```python
from build123d import *

# Parameters (mm, degrees)
SKETCH_2_W           = 70
SKETCH_2_H           = 60
EXTRUDE_2_DEPTH      = 40
SKETCH_3_W           = 40.7
SKETCH_3_H           = 20.5
CUT_EXTRUDE_1_DEPTH  = 28
SKETCH_4_W           = 14.65
SKETCH_4_H           = 20.5
EXTRUDE_3_DEPTH      = 28
SKETCH_15_W          = 40.7
SKETCH_15_H          = 40.25
CUT_EXTRUDE_6_DEPTH  = 28
SKETCH_16_W          = 14.65
SKETCH_16_H          = 20.204149113
CUT_EXTRUDE_7_DEPTH  = 40
M3X0_5_2_D           = 2.5
CUT_EXTRUDE_8_DEPTH  = 3
CUT_EXTRUDE_9_DEPTH  = 3
CUT_EXTRUDE_10_DEPTH = 6
M3X0_5_3_D           = 2.5
M3X0_5_3_DEPTH       = 40
M3X0_5_3_TIP         = 0.751075774
CUT_EXTRUDE_12_DEPTH = 5


with BuildPart() as part:
    # ｽｹｯﾁ2 → ﾎﾞｽ - 押し出し2 (new body)
    with BuildSketch(Plane.XY):
        Rectangle(SKETCH_2_W, SKETCH_2_H)
    extrude(amount=EXTRUDE_2_DEPTH)

    # ｽｹｯﾁ3 → ｶｯﾄ - 押し出し1 (cut)
    with BuildSketch(Plane.XY):
        Rectangle(SKETCH_3_W, SKETCH_3_H)
    extrude(amount=CUT_EXTRUDE_1_DEPTH, mode=Mode.SUBTRACT)

    # ｽｹｯﾁ4 → ﾎﾞｽ - 押し出し3 (add)
    with BuildSketch(Plane.XY):
        with Locations((27.675, 0)):
            Rectangle(SKETCH_4_W, SKETCH_4_H)
    extrude(amount=EXTRUDE_3_DEPTH)

    # ｽｹｯﾁ15 → ｶｯﾄ - 押し出し6 (cut)
    with BuildSketch(Plane.XY):
        with Locations((0, -9.875)):
            Rectangle(SKETCH_15_W, SKETCH_15_H)
    extrude(amount=CUT_EXTRUDE_6_DEPTH, mode=Mode.SUBTRACT)

    # ｽｹｯﾁ16 → ｶｯﾄ - 押し出し7 (cut)
    with BuildSketch(Plane(origin=(0, -30, 0), x_dir=(-1, 0, 0), z_dir=(0, -1, 0))):
        with Locations((-27.675, -17.897925444)):
            Rectangle(SKETCH_16_W, SKETCH_16_H)
    extrude(amount=-CUT_EXTRUDE_7_DEPTH, mode=Mode.SUBTRACT)

    # M3x0.5 ねじ穴2 (through all)
    with Locations(Plane(origin=(0, 0, 0), x_dir=(-1, 0, 0), z_dir=(0, 0, -1))):
        with Locations((24.85, 5), (24.85, -5)):
            m3x0_5_2 = Hole(M3X0_5_2_D / 2)

    # ﾐﾗｰ1: M3x0.5 ねじ穴2 across plane
    add(m3x0_5_2.mirror(Plane(origin=(0, 0, 0), x_dir=(0, 0, 1), z_dir=(1, 0, 0))), mode=Mode.SUBTRACT)

    # ｽｹｯﾁ17 → ｶｯﾄ - 押し出し8 (cut)
    with BuildSketch(Plane.XY.offset(40)):
        Polygon((-24.85, 8.290896534), (-27.7, 6.645448267), (-27.7, 3.354551733), (-24.85, 1.709103466), (-22, 3.354551733), (-22, 6.645448267), align=None)
        Polygon((-22, -6.645448267), (-22, -3.354551733), (-24.85, -1.709103466), (-27.7, -3.354551733), (-27.7, -6.645448267), (-24.85, -8.290896534), align=None)
    extrude(amount=-CUT_EXTRUDE_8_DEPTH, mode=Mode.SUBTRACT)

    # ｽｹｯﾁ18 → ｶｯﾄ - 押し出し9 (cut)
    with BuildSketch(Plane.XY.offset(7.795850887)):
        Polygon((27.7, 3.354551733), (27.7, 6.645448267), (24.85, 8.290896534), (22, 6.645448267), (22, 3.354551733), (24.85, 1.709103466), align=None)
        Polygon((27.7, -6.645448267), (27.7, -3.354551733), (24.85, -1.709103466), (22, -3.354551733), (22, -6.645448267), (24.85, -8.290896534), align=None)
    extrude(amount=-CUT_EXTRUDE_9_DEPTH, mode=Mode.SUBTRACT)

    # ｽｹｯﾁ19 → ｶｯﾄ - 押し出し10 (cut)
    with BuildSketch(Plane(origin=(0, 0, 20), x_dir=(-1, 0, 0), z_dir=(0, 0, -1))):
        Polygon((35, 1.709103466), (35, 8.290896534), (24.85, 8.290896534), (27.7, 6.645448267), (27.7, 3.354551733), (24.85, 1.709103466), align=None)
        Polygon((22, 6.645448267), (22, 3.354551733), (24.85, 1.709103466), (27.7, 3.354551733), (27.7, 6.645448267), (24.85, 8.290896534), align=None)
        Polygon((22, -6.645448267), (24.85, -8.290896534), (27.7, -6.645448267), (27.7, -3.354551733), (24.85, -1.709103466), (22, -3.354551733), align=None)
        Polygon((35, -8.290896534), (24.85, -8.290896534), (27.7, -6.645448267), (27.7, -3.354551733), (24.85, -1.709103466), (35, -1.709103466), align=None)
    extrude(amount=-CUT_EXTRUDE_10_DEPTH, mode=Mode.SUBTRACT)

    # M3x0.5 ねじ穴3
    with Locations(Plane(origin=(35, 0, 0), x_dir=(0, 0, -1), z_dir=(1, 0, 0))):
        with Locations((-4, -20), (-36, -20), (-10, 20), (-30, 20)):
            Hole(M3X0_5_3_D / 2, depth=M3X0_5_3_DEPTH)
            with Locations((0, 0, -(M3X0_5_3_DEPTH + M3X0_5_3_TIP / 2))):  # 118° drill point
                Cone(0, M3X0_5_3_D / 2, M3X0_5_3_TIP, mode=Mode.SUBTRACT)

    # ｽｹｯﾁ24 → ｶｯﾄ - 押し出し12 (cut)
    with BuildSketch(Plane(origin=(20, 0, 0), x_dir=(0, 0, -1), z_dir=(1, 0, 0))):
        Polygon((-38.85, -18.354551733), (-38.85, -21.645448267), (-36, -23.290896534), (-33.15, -21.645448267), (-33.15, -18.354551733), (-36, -16.709103466), align=None)
        Polygon((-40, -16.709103466), (-40, -23.290896534), (-36, -23.290896534), (-38.85, -21.645448267), (-38.85, -18.354551733), (-36, -16.709103466), align=None)
        Polygon((-6.85, -18.354551733), (-6.85, -21.645448267), (-4, -23.290896534), (-1.15, -21.645448267), (-1.15, -18.354551733), (-4, -16.709103466), align=None)
        Polygon((-10, 23.290896534), (-7.15, 21.645448267), (-7.15, 30), (-12.85, 30), (-12.85, 21.645448267), align=None)
        Polygon((-12.85, 21.645448267), (-12.85, 18.354551733), (-10, 16.709103466), (-7.15, 18.354551733), (-7.15, 21.645448267), (-10, 23.290896534), align=None)
        Polygon((-32.85, 21.645448267), (-32.85, 18.354551733), (-30, 16.709103466), (-27.15, 18.354551733), (-27.15, 21.645448267), (-30, 23.290896534), align=None)
        Polygon((-30, 23.290896534), (-27.15, 21.645448267), (-27.15, 30), (-32.85, 30), (-32.85, 21.645448267), align=None)
        Polygon((0, -23.290896534), (0, -16.709103466), (-4, -16.709103466), (-1.15, -18.354551733), (-1.15, -21.645448267), (-4, -23.290896534), align=None)
    extrude(amount=-CUT_EXTRUDE_12_DEPTH, mode=Mode.SUBTRACT)


solid = part.part
```
Work out the finished part from the listing and answer in its coordinate system (mm). A direction names the side the tool comes from. Round coordinates to 2 decimals unless told otherwise and drop trailing zeros. Write each loop counter-clockwise with the first axis right and the second up, starting at its lowest first coordinate (ties: lowest second). Pieces come first, ordered by that corner, then holes.
1) A cutting plane is placed at A-A on y = 25.5. Determine the outline of the cut face in (x, z), and give its area (3 significant figures).
2) Flat-ended cylindrical pins translate along their axes: P1, Ø3, axis at y = -6, z = 23, coming from the +X side; P2, Ø3, axis at x = -24.85, y = -5, coming from the +Z side. Find the tip coordinate at first contact, or state that the pin passes through.
3) Determine the mould class of faces 1 (the face through (-22, -5, 23)), 2 (the face through (-24.9, -6.4, 37)), 3 (the face through (0, 14, 0)) for opening direction X: pulls with the +X half, pulls with the -X half, needs draft (parallel to the pull), parting line crosses it, or undercut.
4) Which of the six approach directions +Z, -Z, +X, -X, +Y, -Y give full straight-line access (tool end or side, diameter ignored) to faces 4 (the face through (0, 10.25, 14)), 5 (the face through (-23.41, 2.54, 22.96)), 6 (the face through (27.39, -20.76, 35.01)), 7 (the face through (-22, 5, 39))?
5) A cutting plane is placed at D-D on x = 17. Determine the outline of the cut face in (y, z).
6) Consider probe 1 along X at (y, z) = (-5, 37.75); probe 2 along Z at (x, y) = (3, 20); probe 3 along Y at (x, z) = (4, 10). Determine where each line is inside the solid, lowest interval first.
7) A cutting plane is placed at C-C on y = -5. Give the number of separate pieces and of enclosed holes in the cut face, and give its area (3 significant figures).
8) A cutting plane is placed at B-B on x = -8.5. Determine the outline of the cut face in (y, z), and give its area (3 significant figures).
Entries:
1. outline: (-35, 0) - (35, 0) - (35, 40) - (-35, 40) - close; hole (15, 7.15) - (20, 7.15) - (20, 12.85) - (15, 12.85) - close; hole (15, 27.15) - (20, 27.15) - (20, 32.85) - (15, 32.85) - close
1. area: 2,740 mm2
2. P1: stops at x = -20.35
2. P2: stops at z = 37
3. face 1: pulls with the -X half
3. face 2: undercut
3. face 3: needs draft
4. face 4: -Z, -Y
4. face 5: -X
4. face 6: +X
4. face 7: +Z
5. outline: (-30, 28) - (10.25, 28) - (10.25, 0) - (30, 0) - (30, 7.15) - (18.35, 7.15) - (16.71, 10) - (18.35, 12.85) - (30, 12.85) - (30, 27.15) - (18.35, 27.15) - (16.71, 30) - (18.35, 32.85) - (30, 32.85) - (30, 40) - (-16.71, 40) - (-16.71, 36) - (-18.35, 33.15) - (-21.65, 33.15) - (-23.29, 36) - (-23.29, 40) - (-30, 40) - close
6. probe 1: x = -35 to -27.7, -22 to 23.6, 26.1 to 35
6. probe 2: z = 0 to 8.75, 11.25 to 28.75, 31.25 to 40
6. probe 3: y = 10.25 to 18.75, 21.25 to 30
7. separate pieces: 6
7. enclosed holes: 0
7. area: 1,130 mm2
8. outline: (-30, 28) - (10.25, 28) - (10.25, 0) - (30, 0) - (30, 40) - (-30, 40) - close
8. area: 1,270 mm2
